from build123d import *

# Parameters (mm, degrees)
SKETCH1_W           = 55
SKETCH1_H           = 18.5
BOSS_EXTRUDE1_DEPTH = 9
SKETCH2_W           = 37
SKETCH2_H           = 18.5
BOSS_EXTRUDE2_DEPTH = 10
SKETCH3_W           = 4
SKETCH3_H           = 19
BOSS_EXTRUDE3_DEPTH = 4
SKETCH4_W           = 11.25
SKETCH4_H           = 10
BOSS_EXTRUDE4_DEPTH = 30


with BuildPart() as part:
    # Sketch1 → Boss-Extrude1 (new body)
    with BuildSketch(Plane(origin=(0, 0, 0), x_dir=(1, 0, 0), z_dir=(0, 1, 0))):
        Rectangle(SKETCH1_W, SKETCH1_H)
    extrude(amount=BOSS_EXTRUDE1_DEPTH)

    # Sketch2 → Boss-Extrude2 (add)
    with BuildSketch(Plane(origin=(0, 9, 0), x_dir=(1, 0, 0), z_dir=(0, 1, 0))):
        with Locations((-9, 0)):
            Rectangle(SKETCH2_W, SKETCH2_H)
    extrude(amount=BOSS_EXTRUDE2_DEPTH)

    # Sketch3 → Boss-Extrude3 (add)
    with BuildSketch(Plane.ZY.offset(27.5)):
        with Locations((0, 9.5)):
            Rectangle(SKETCH3_W, SKETCH3_H)
    extrude(amount=BOSS_EXTRUDE3_DEPTH)

    # Sketch4 → Boss-Extrude4 (add)
    with BuildSketch(Plane.ZY.offset(27.5)):
        with Locations((3.625, 14)):
            Rectangle(SKETCH4_W, SKETCH4_H)
    extrude(amount=BOSS_EXTRUDE4_DEPTH)


solid = part.part
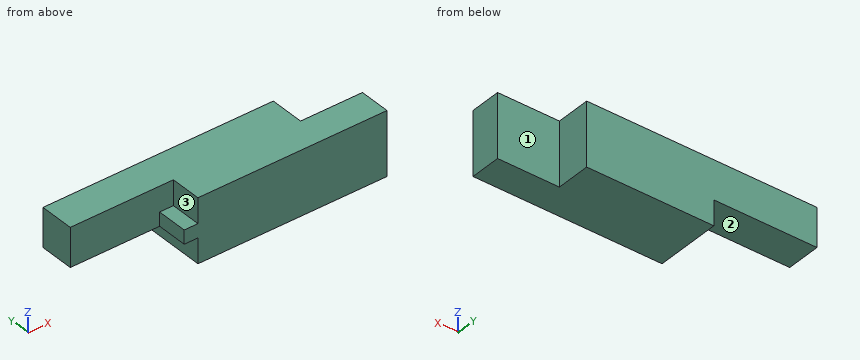
For this review, take the finished solid that the model builds, in its own axes (mm). Face numbers are marked on the shaded views. A direction names the side the tool comes from. Round coordinates to 2 decimals unless told otherwise and drop trailing zeros. Write each loop counter-clockwise with the first axis right and the second up, starting at its lowest first coordinate (ties: lowest second). Pieces come first, ordered by that corner, then holes. Notation, with made-up numbers: (37.25, 28) - (95.25, 28) arc R27 cw to (95.25, 63) - close; hole circle Ø11 at (18.5, 14). An arc over 180 degrees is marked (long way). Write item = value, one per line. Start each with the question number.
1. For pin 1 Ø3 at (y, z) = (12.5, 0) entering from +X; pin 2 Ø3 at (x, y) = (12.5, 12.5) entering from +Z; pin 3 Ø3.5 at (y, z) = (4, 5) entering from -X; pin 4 Ø10 at (x, y) = (-43.5, 11.5) entering from -Z, all flat-tipped, find the tip position at first contact; note any pin that passes through.
2. For the marked faces 1, 2 and 3, list the 3-axis set-ups (+Z, -Z, +X, -X, +Y, -Y) from which the entire face can be reached by the end or side of a thin tool; tool diameter is ignored.
3. Consider section A-A on z = 0.75. State the section outline as (x, y) points, plus the area to 3 significant figures.
4. Consider section B-B on y = 5.25. State the section outline as (x, z) points, plus the area to 3 significant figures.
5. Wall thickness on L1, parallel to Y at x = 20.5, z = 5.5; L2, parallel to X at y = 10.75, z = 2; L3, parallel to X at y = 5.5, z = 3.5: over which ranges is each line inside the solid? List them lowest first.
6. Consider section C-C on x = -44. State the section outline as (y, z) points.
7. Consider section D-D on z = -3.75. State the section outline as (x, y) points.
Evaluation:
q1.pin_1 = 9.5
q1.pin_2 = through
q1.pin_3 = -27.5
q1.pin_4 = -2
q2.face_1 = +Z, -Z, +X, +Y
q2.face_2 = -Z, -X, +Y, -Y
q2.face_3 = +Z, -X, -Y
q3.outline = (-57.5, 9) - (-31.5, 9) - (-31.5, 0) - (27.5, 0) - (27.5, 9) - (9.5, 9) - (9.5, 19) - (-57.5, 19) - close
q3.area = 1,200 mm2
q4.outline = (-31.5, -2) - (-27.5, -2) - (-27.5, -9.25) - (27.5, -9.25) - (27.5, 9.25) - (-27.5, 9.25) - (-27.5, 2) - (-31.5, 2) - close
q4.area = 1,030 mm2
q5.L1 = 0 to 9
q5.L2 = -57.5 to 9.5
q5.L3 = -27.5 to 27.5
q6.outline = (9, -2) - (19, -2) - (19, 9.25) - (9, 9.25) - close
q7.outline = (-27.5, 0) - (27.5, 0) - (27.5, 9) - (9.5, 9) - (9.5, 19) - (-27.5, 19) - close
